Design review of the part built by this model. Coordinates are the model's own, in mm. Face numbers are marked on the shaded views. A direction names the side the tool comes from. Give positions to 0.01 mm unless a question says otherwise; leave off trailing zeros. Write each loop counter-clockwise with the first axis right and the second up, starting at its lowest first coordinate (ties: lowest second). Pieces come first, ordered by that corner, then holes. Notation, with made-up numbers: (-20.75, 58.5) -> (26.25, 58.5) arc R19 ccw to (26.25, 63.5) -> close; hole circle Ø11 at (1, -23.75). An arc over 180 degrees is marked (long way). Use CSV: the item, a comma, the result in double quotes.
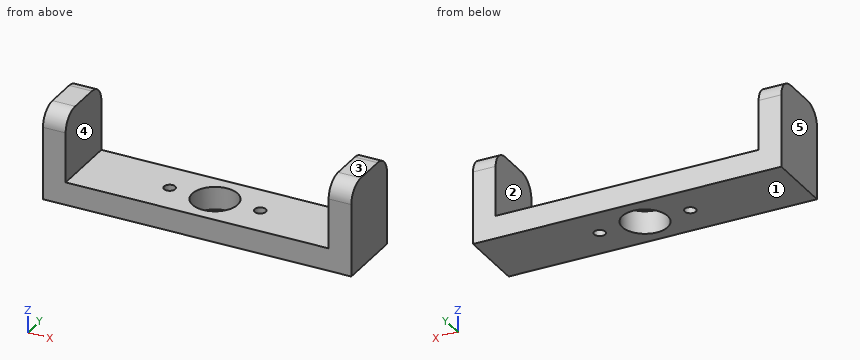
Autodesk Fusion 360 part; units mm, degrees
sketch "Sketch1" plane through (0, 0, 0) normal (0, 0, 1) x (1, 0, 0)
  line L0 (34, -7.5) -> (-34, -7.5)
  line L1 (-34, -7.5) -> (-34, 7.5)
  line L2 (-34, 7.5) -> (34, 7.5)
  line L3 (34, 7.5) -> (34, -7.5)
  line L4 (34, -7.5) -> (-34, 7.5) construction
  line L5 (-34, -7.5) -> (34, 7.5) construction
  circle A0 centre (0, 0) radius 5
  line L6 (0, 0) -> (10, 0) construction
  circle A1 centre (10, 0) radius 1.25
  line L7 (0, 2.5) -> (0, 20)
  circle A2 centre (-10, 0) radius 1.25
  dimension "d18" = 68
  dimension "d19" = 15
  dimension "d20" = 10
  dimension "d22" = 10
  dimension "d23" = 2.5
extrude "Extrude1" add sketch "Sketch1" along normal blind 5
sketch "Sketch2" plane through (0, 0, 5) normal (0, 0, 1) x (-1, 0, 0)
  line L0 (0, -2.5) -> (0, -20)
  circle A0 centre (-10, 0) radius 1.25
  circle A1 centre (10, 0) radius 1.25
  circle A2 centre (0, 0) radius 5
  line L1 (-34, -7.5) -> (34, -7.5)
  line L2 (34, -7.5) -> (34, 7.5)
  line L3 (34, 7.5) -> (-34, 7.5)
  line L4 (-34, 7.5) -> (-34, -7.5)
  line L5 (34, -7.5) -> (29, -7.5)
  line L6 (29, -7.5) -> (29, 7.5)
  line L7 (29, 7.5) -> (34, 7.5)
  line L8 (34, 7.5) -> (34, -7.5)
  line L9 (-34, -7.5) -> (-29, -7.5)
  line L10 (-29, -7.5) -> (-29, 7.5)
  line L11 (-29, 7.5) -> (-34, 7.5)
  line L12 (-34, 7.5) -> (-34, -7.5)
  dimension "d24" = 5
  dimension "d25" = 5
extrude "Extrude2" add sketch "Sketch2" along normal blind 15 contours L1 L3 L4 L9 L10 L11 L12 | L1 L2 L3 L5 L6 L7 L8
fillet "Fillet2" radius 4 4 edges at (-31.5, -7.5, 20) (-31.5, 7.5, 20) (31.5, -7.5, 20) (31.5, 7.5, 20)
(1) Take a section at D-D (z = 1.75). Write out the cut boundary in (x, y), then the cut area to 3 significant figures.
Established:
outline,"(-34, -7.5) -> (34, -7.5) -> (34, 7.5) -> (-34, 7.5) -> close; hole circle Ø2.5 at (-10, 0); hole circle Ø10 at (0, 0); hole circle Ø2.5 at (10, 0)"
area,"932 mm2"
(2) For line 1 along X through (y, z) = (1.25, 15.5); line 2 along Y through (x, z) = (-10, 3.4); line 3 along Y through (x, z) = (0, 2.5), list the stretches that pass through material, from the lowest coordinate up. Write a range as [from, to].
Established:
line 1,"x = [-34, -29], [29, 34]"
line 2,"y = [-7.5, -1.25], [1.25, 7.5]"
line 3,"y = [-7.5, -5], [5, 7.5]"
(3) Take a section at A-A (y = 0). Write out the cut boundary in (x, z), then the cut area to 3 significant figures.
Established:
outline,"(-34, 0) -> (-11.25, 0) -> (-11.25, 5) -> (-29, 5) -> (-29, 20) -> (-34, 20) -> close; (-8.75, 0) -> (-5, 0) -> (-5, 5) -> (-8.75, 5) -> close; (5, 0) -> (8.75, 0) -> (8.75, 5) -> (5, 5) -> close; (11.25, 0) -> (34, 0) -> (34, 20) -> (29, 20) -> (29, 5) -> (11.25, 5) -> close"
area,"415 mm2"
(4) Clearance check with flat-ended pins moving along their axes: pin 1 (1 mm diameter, centred on x = -18, y = -5, fed in from -Z); pin 2 (1.5 mm diameter, centred on x = 5, y = 1, fed in from +Z). State where each tip first meets the part, or that it passes through.
Established:
pin 1,"stops at z = 0"
pin 2,"stops at z = 5"
(5) Mouldability with a two-part tool opening along X and no side actions: class the marked faces 3, 4 and 5 as +X half, -X half, draft (parallel to the pull), parting line (faces both ways), or undercut.
Established:
face 3,"draft"
face 4,"undercut"
face 5,"-X half"
(6) Tool access review of the marked faces 1 and 2: name each direction out of +Z, -Z, +X, -X, +Y, -Y from which nothing blocks a thin tool from reaching the whole face with its end or side.
Established:
face 1,"-Z, +X, -X, +Y, -Y"
face 2,"+Z, +Y, -Y"
(7) Take a section at C-C (z = 8.5). Write out the cut boundary in (x, y).
Established:
outline,"(-34, -7.5) -> (-29, -7.5) -> (-29, 7.5) -> (-34, 7.5) -> close; (29, -7.5) -> (34, -7.5) -> (34, 7.5) -> (29, 7.5) -> close"
(8) Take a section at B-B (x = 0). Write out the cut boundary in (y, z).
Established:
outline,"(-7.5, 0) -> (-5, 0) -> (-5, 5) -> (-7.5, 5) -> close; (5, 0) -> (7.5, 0) -> (7.5, 5) -> (5, 5) -> close"
